```python
from build123d import *


with BuildPart() as part:
    # Sketch1 → Revolve1 (revolve)
    with BuildSketch(Plane(origin=(0, 0, 0), x_dir=(1, 0, 0), z_dir=(0, 1, 0)), mode=Mode.PRIVATE) as revolve1_sk:
        Polygon((-73.661954618, 36), (-25.262429889, 36), (-11.25804845, 11.743699818), (-9.154700538, 11.743699818), (-8, 13.743699818), (0, 13.743699818), (0, 4.225), (-9.8, 4.225), (-11.661954618, 1), (-13.661954618, 1), (-13.661954618, 1.6), (-23.661954618, 1.6), (-23.661954618, 24.75), (-32.661954618, 33.75), (-73.661954618, 33.75), align=None)
    revolve(revolve1_sk.sketch.rotate(Axis((-73.661954618, 0, 0), (1, 0, 0)), 180), axis=Axis((-73.661954618, 0, 0), (1, 0, 0)))


solid = part.part
```
Verification items for the finished model (mm, model axes). A direction names the side the tool comes from. Coordinates: 2 decimals unless noted, no trailing zeros. Order: outer loops, then holes, each group sorted by start corner. A loop starts at its lowest first (then second) coordinate and runs counter-clockwise, first axis right, second up. Notation, with made-up numbers: (-30.75, 67.25) - (5.25, 67.25) arc R14 ccw to (5.25, 73.25) - close; hole circle Ø2 at (79.25, 60.5). An arc over 180 degrees is marked (long way). Return JSON: item names as keys, results as strings.
(1) Thickness scan on line 1 along Y through (x, z) = (-7, 0) (3 decimals); line 2 along Y through (x, z) = (-62, 0); line 3 along X through (y, z) = (8.5, -7.5). Record the ranges inside material, lowest first.
Filled sheet:
{"line 1": "y = -13.744 to -4.225, 4.225 to 13.744", "line 2": "y = -36 to -33.75, 33.75 to 36", "line 3": "x = -23.66 to 0"}
(2) Mould release check, pull along Z, two halves, no side actions. Record for faces 1 (the flat face through (-13.662, 1, 1)), 2 (the conical face through (-11.938, -3.881, 12.325)), 3 (the flat face through (-73.662, -10.8, 32.2)): pulls with the +Z half, pulls with the -Z half, needs draft (parallel to the pull), parting line crosses it, or undercut.
Filled sheet:
{"face 1": "undercut", "face 2": "parting line crosses it", "face 3": "needs draft"}
(3) Section check B-B, the plane x = -20.5. Record the cut outline in (y, z).
Filled sheet:
{"outline": "circle Ø55.5 at (0, 0); hole circle Ø3.2 at (0, 0)"}
(4) Go/stop test with flat-tipped pins: pin 1 (1.5 mm diameter, centred on y = -14.5, z = 3, fed in from +X); pin 2 (2.5 mm diameter, centred on y = 0, z = 0, fed in from -X); pin 3 (3 mm diameter, centred on x = -48.5, z = 10, fed in from -Y). Record where each tip stops, or that it passes through.
Filled sheet:
{"pin 1": "stops at x = -12.59", "pin 2": "stops at x = -13.66", "pin 3": "stops at y = -34.98"}
(5) Section check A-A, the plane x = -58.5. Record the cut outline in (y, z), and give its area (3 significant figures).
Filled sheet:
{"outline": "circle Ø72 at (0, 0); hole circle Ø67.5 at (0, 0)", "area": "493 mm^2"}
(6) Access from +Z, -Z, +X, -X, +Y, -Y to the whole of each face (thin tool, end or side, straight path). Record for faces 4 (the cylindrical face through (-10.19, -3.53, 11.2)), 5 (the cylindrical face through (-4.97, -1.27, 4.03)), 6 (the cylindrical face through (-53.449, 32.947, -7.316)).
Filled sheet:
{"face 4": "none", "face 5": "+X", "face 6": "-X"}
